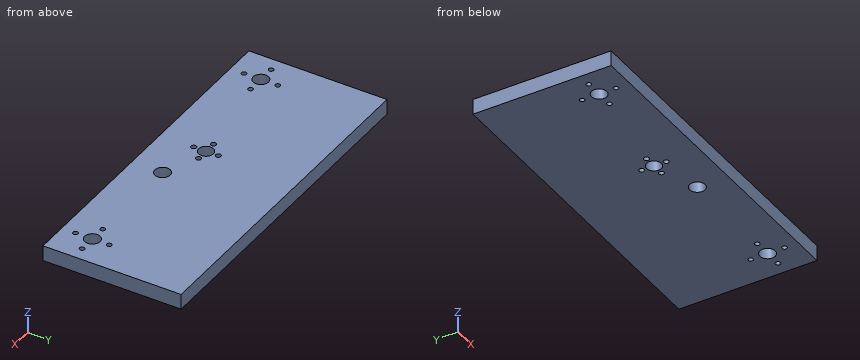
Solid Edge part; units mm, degrees
sketch "Sketch1" plane through (0, 0, 0) normal (0, 0, 1) x (1, 0, 0)
  line L0 (-110, -40) -> (110, -40)
  line L1 (110, -40) -> (110, 40)
  line L2 (110, 40) -> (-110, 40)
  line L3 (-110, 40) -> (-110, -40)
  dimension "D1" = 110
  dimension "D2" = 110
extrude "Protrusion1" add sketch "Sketch1" along normal blind 10
sketch "Sketch2" plane through (0, -40, 5) normal (0, -1, 0) x (1, 0, 0)
  line L0 (-110, 5) -> (110, 5)
  line L1 (110, 5) -> (110, -5)
  line L2 (110, -5) -> (-110, -5)
  line L3 (-110, -5) -> (-110, 5)
extrude "Extrusionsausprägung_2" add sketch "Sketch2" along normal blind 10
sketch "Sketch3" plane through (0, -5, 10) normal (0, 0, 1) x (1, 0, 0)
  circle A0 centre (-90, -25) radius 5
  dimension "D1" = 90
extrude "Cutout1" cut sketch "Sketch3" against normal up to next
hole "Bohrung_2" at (-90, -19, 10) direction (0, 0, -1) diameter 3.2 end up to next
hole "Hole1" at (-101, -30, 10) direction (0, 0, -1) diameter 3.2 end up to next
hole "Hole2" at (-90, -41, 10) direction (0, 0, -1) diameter 3.2 end up to next
hole "Hole3" at (-79, -30, 10) direction (0, 0, -1) diameter 3.2 end up to next
mirror "Mirror1" about plane through (0, 0, 0) normal (1, 0, 0) of "Cutout1", "Bohrung_2", "Hole1", "Hole2", "Hole3"
sketch "Sketch4" plane through (0, -5, 10) normal (0, 0, 1) x (1, 0, 0)
  circle A0 centre (15, -25) radius 5
extrude "Cutout2" cut sketch "Sketch4" against normal up to next
sketch "Sketch5" plane through (0, -5, 10) normal (0, 0, 1) x (1, 0, 0)
  circle A0 centre (-15, -15) radius 4.8361
  circle A1 centre (-15, -7) radius 1.7
  circle A2 centre (-7, -15) radius 1.7
  circle A3 centre (-15, -23) radius 1.7
  circle A4 centre (-23, -15) radius 1.7
  dimension "D1" = 15
extrude "Cutout3" cut sketch "Sketch5" against normal up to next
properties material "Nylon, allgemein"
Work out the finished part from the listing and answer in its coordinate system (mm). Round coordinates to 2 decimals unless told otherwise and drop trailing zeros. Loops run counter-clockwise (first coordinate to the right, second up) from the corner with the lowest first, then second, coordinate; pieces in that order, holes last. Notation, with made-up numbers: (26, 43.25) -> (34, 43.25) arc R26 ccw to (34, 61.25) -> close; hole circle Ø5 at (-5.75, 89). An arc over 180 degrees is marked (long way). Write each question's results on one line, items separated by ' | '. Start each with the question number.
1. Find the intervals of material crossed by probe 1 along X at (y, z) = (-41, 4); probe 2 along Y at (x, z) = (-15, 6.5); probe 3 along Y at (x, z) = (90, 2.5), in increasing order. Write a range as from..to.
2. Section B-B (z = 6.25) is taken. State how many separate pieces and enclosed holes the cut face has, plus the area to 3 significant figures.
3. Section A-A (x = 15) is taken. Determine the outline of the cut face in (y, z).
Evaluation:
1) probe 1: x = -110..-91.6, -88.4..88.4, 91.6..110 | probe 2: y = -50..-29.7, -26.3..-24.84, -15.16..-13.7, -10.3..40 | probe 3: y = -50..-42.6, -39.4..-35, -25..-20.6, -17.4..40
2) separate pieces: 1 | enclosed holes: 16 | area: 19,400 mm2
3) outline: (-50, 0) -> (-35, 0) -> (-35, 10) -> (-50, 10) -> close; (-25, 0) -> (40, 0) -> (40, 10) -> (-25, 10) -> close
